Could you check a few things on this model? Use its own coordinates, in mm. A direction names the side the tool comes from. Round coordinates to 2 decimals unless told otherwise and drop trailing zeros. Write each loop counter-clockwise with the first axis right and the second up, starting at its lowest first coordinate (ties: lowest second). Pieces come first, ordered by that corner, then holes. Notation, with made-up numbers: (16, 15.5) -> (35, 15.5) arc R33 cw to (35, 51.5) -> close; hole circle Ø4 at (-30.75, 27.25). An arc over 180 degrees is marked (long way). Return JSON: item names as keys, results as strings.
Autodesk Fusion 360 part; units mm, degrees
sketch "Sketch1" plane through (0, 0, 0) normal (0, 0, 1) x (1, 0, 0)
  line L0 (25, 42.5) -> (-25, 42.5)
  line L1 (-25, 42.5) -> (-25, -42.5)
  line L2 (-25, -42.5) -> (25, -42.5)
  line L3 (25, -42.5) -> (25, 42.5)
  line L4 (25, 42.5) -> (-25, -42.5) construction
  line L5 (-25, 42.5) -> (25, -42.5) construction
  line L6 (25, 42.5) -> (46.6506, 55)
  line L7 (25, 42.5) -> (55, 42.5) construction
  line L8 (0, 42.5) -> (0, -42.5)
  line L9 (-25, 0) -> (25, 0)
  line L10 (25, 42.5) -> (23.5, 45.0981)
  line L11 (23.5, 45.0981) -> (45.1506, 57.5981)
  line L12 (45.1506, 57.5981) -> (46.6506, 55)
  line L13 (25, 42.5) -> (26.5, 39.9019)
  line L14 (26.5, 39.9019) -> (48.1506, 52.4019)
  line L15 (23.5, 45.0981) -> (19, 42.5)
  line L16 (26.5, 39.9019) -> (25, 39.0359)
  line L17 (48.1506, 52.4019) -> (46.6506, 55)
  circle A0 centre (46.6506, 55) radius 8.75
  circle A1 centre (46.6506, 55) radius 7.75
  line L18 (46.6506, 55) -> (42.7756, 61.7117)
  line L19 (46.6506, 55) -> (53.3623, 58.875)
  line L20 (46.6506, 55) -> (50.5256, 48.2883)
  circle A2 centre (46.6506, 55) radius 1.5
  line L21 (46.6506, 55) -> (50.9808, 57.5)
  circle A3 centre (50.9808, 57.5) radius 1.1
  circle A4 centre (42.3205, 52.5) radius 1.1
  line L22 (46.6506, 55) -> (44.1506, 59.3301)
  circle A5 centre (44.1506, 59.3301) radius 1.1
  circle A6 centre (49.1506, 50.6699) radius 1.1
  circle A7 centre (-49.1506, 50.6699) radius 1.1
  circle A8 centre (-50.9808, 57.5) radius 1.1
  circle A9 centre (-44.1506, 59.3301) radius 1.1
  circle A10 centre (-46.6506, 55) radius 1.5
  circle A11 centre (-42.3205, 52.5) radius 1.1
  line L23 (-23.5, 45.0981) -> (-45.1506, 57.5981)
  line L24 (-26.5, 39.9019) -> (-48.1506, 52.4019)
  circle A12 centre (-46.6506, 55) radius 8.75
  circle A13 centre (-46.6506, 55) radius 7.75
  line L25 (-26.5, 39.9019) -> (-25, 39.0359)
  line L26 (-23.5, 45.0981) -> (-19, 42.5)
  circle A14 centre (-46.6506, -55) radius 7.75
  circle A15 centre (-44.1506, -59.3301) radius 1.1
  circle A16 centre (-46.6506, -55) radius 1.5
  circle A17 centre (-49.1506, -50.6699) radius 1.1
  circle A18 centre (-42.3205, -52.5) radius 1.1
  circle A19 centre (-50.9808, -57.5) radius 1.1
  line L27 (-26.5, -39.9019) -> (-48.1506, -52.4019)
  line L28 (-23.5, -45.0981) -> (-45.1506, -57.5981)
  line L29 (-23.5, -45.0981) -> (-19, -42.5)
  line L30 (-26.5, -39.9019) -> (-25, -39.0359)
  line L31 (23.5, -45.0981) -> (19, -42.5)
  line L32 (26.5, -39.9019) -> (25, -39.0359)
  line L33 (26.5, -39.9019) -> (48.1506, -52.4019)
  line L34 (23.5, -45.0981) -> (45.1506, -57.5981)
  circle A20 centre (46.6506, -55) radius 8.75
  circle A21 centre (46.6506, -55) radius 7.75
  circle A22 centre (49.1506, -50.6699) radius 1.1
  circle A23 centre (46.6506, -55) radius 1.5
  circle A24 centre (42.3205, -52.5) radius 1.1
  circle A25 centre (44.1506, -59.3301) radius 1.1
  circle A26 centre (50.9808, -57.5) radius 1.1
  circle A27 centre (-46.6506, -55) radius 7.75
  circle A28 centre (-46.6506, -55) radius 8.75
  line L35 (25, 0) -> (25, -42.5)
  line L36 (0, 0) -> (0, -9)
  line L37 (0, -9) -> (0, -10.6)
  line L38 (0, -9) -> (0, -7.4)
  line L39 (0, -9) -> (1, -9)
  line L40 (19, -42.5) -> (25.9282, -46.5)
  line L41 (25, -39.0359) -> (25.0866, -34.0366)
  line L42 (19, -42.5) -> (16, -42.5)
  line L43 (19, -42.5) -> (14.6699, -40)
  line L44 (14.6699, -40) -> (34.8771, -40) construction
  line L45 (25, -39.0359) -> (17.5453, -34.8631)
  line L46 (14.6699, -40) -> (17.5453, -34.8631)
  line L47 (17.5453, -34.8631) -> (25, -21.5453)
  line L48 (25, -42.5) -> (25, -33)
  line L49 (25, -33) -> (15.5, -33)
  circle A29 centre (15.5, -33) radius 2.3
  circle A30 centre (15.5, -33) radius 4
  line L50 (-25, -42.5) -> (-18, -42.5)
  line L51 (-18, -42.5) -> (-18, -27.5)
  line L52 (-18, 42.5) -> (-18, 27.5)
  line L53 (-25, 42.5) -> (-18, 42.5)
  line L54 (18, 42.5) -> (18, 27.5)
  line L55 (18, -42.5) -> (18, -27.5)
  line L56 (18, -30) -> (18, 27.5)
  line L57 (18, 27.5) -> (-18, 27.5)
  line L58 (-18, 27.5) -> (-18, -27.5)
  line L59 (18, -27.5) -> (-18, -27.5)
  circle A31 centre (15.5, -33) radius 1.25
  circle A32 centre (-15.5, -33) radius 1.25
  circle A33 centre (-15.5, -33) radius 2.3
  circle A34 centre (-15.5, -33) radius 4
  circle A35 centre (-15.5, 33) radius 4
  circle A36 centre (-15.5, 33) radius 2.3
  circle A37 centre (-15.5, 33) radius 1.25
  circle A38 centre (15.5, 33) radius 1.25
  circle A39 centre (15.5, 33) radius 2.3
  circle A40 centre (15.5, 33) radius 4
  line L60 (18, 27.5) -> (18, 15.5)
  line L61 (18, 15.5) -> (-18, 15.5)
  line L62 (18, 15.5) -> (18, 10.5)
  line L63 (18, 10.5) -> (-18, 10.5)
  line L64 (18, -10.5) -> (-18, -10.5)
  line L65 (18, -15.5) -> (-18, -15.5)
  line L66 (0, 0) -> (0, 2.5)
  line L67 (0, 2.5) -> (-18, 2.5)
  line L68 (0, 2.5) -> (18, 2.5)
  line L69 (0, -2.5) -> (18, -2.5)
  line L70 (0, -2.5) -> (-18, -2.5)
  line L71 (0, 27.5) -> (10, 27.5)
  line L72 (10, 27.5) -> (10, 42.5)
  line L73 (-10, 27.5) -> (-10, 42.5)
  line L74 (10, 42.5) -> (10, 35.5)
  line L75 (10, 35.5) -> (-10, 35.5)
  line L76 (10, -35.5) -> (-10, -35.5)
  line L77 (-10, -27.5) -> (-10, -42.5)
  line L78 (10, -27.5) -> (10, -42.5)
  point P0 (-46.6506, -55)
  dimension "d1" = 50
  dimension "d2" = 85
  dimension "d4" = 25
  dimension "d5" = 30
  dimension "d6" = 3
  dimension "d7" = 25
  dimension "d8" = 17.5
  dimension "d9" = 15.5
  dimension "d10" = 3
  dimension "d11" = 5
  dimension "d12" = 2.2
  dimension "d13" = 5
  dimension "d14" = 2.2
  dimension "d23" = 9
  dimension "d24" = 1.6
  dimension "d25" = 1.6
  dimension "d51" = 8
  dimension "d76" = 5
  dimension "d77" = 3
  dimension "d88" = 5
  dimension "d130" = 180
  dimension "d131" = 9.5
  dimension "d132" = 9.5
  dimension "d133" = 4.6
  dimension "d134" = 8
  dimension "d141" = 7
  dimension "d142" = 15
  dimension "d170" = 2.5
  dimension "d180" = 12
  dimension "d181" = 5
  dimension "d182" = 2.5
  dimension "d186" = 10
  dimension "d187" = 7
extrude "Extrude1" add sketch "Sketch1" along normal blind 2 contours L3 L9 L35 L47 A30 L55 L56 | L3 L35 L47 L49 A30 | L8 L9 L36 L56 L69 | L8 L9 L56 L66 L68 | L3 L35 L45 L48 L49 A30 | L47 L49 A30 | L47 L49 A30 L55 L56 | L8 L36 L37 L38 L56 L64 L69 | L2 L3 L35 L43 L45 L48 A30 L55 | L45 L47 L49 A30 L55 | L47 L49 L55 | L46 L47 A30 L55 L56 | L2 L42 L43 L46 A30 L55 L56 L59 L78 | L8 L37 L56 L64 L65 | L45 A30 L55 | L45 L47 L55 | L43 L46 A30 L55 | L45 L46 A30 L55 | L8 L56 L59 L65 | L2 L42 L43 L55 | L8 L59 L76 L78 | L2 L8 L76 L78
extrude "Extrude3" add sketch "Sketch1" along normal blind 24 contours L47 L49 A30 | L47 L49 A30 L55 L56 | L45 L47 L49 A30 L55 | L47 L49 L55 | A29 | L46 L47 A30 L55 L56 | L45 A30 L55 | L45 L47 L55 | L45 L46 A30 L55
mirror "Mirror3" about plane through (0, -27.5, 0) normal (-1, 0, 0) of bodies 1 merged
extrude "Extrude6" cut sketch "Sketch1" along normal blind 12 contours L8 L36 L37 L38 L56 L64 L69 | L8 L56 L63 L68 | L8 L56 L57 L60 L61 L71 | L8 L58 L63 L67 | L8 L36 L37 L38 L58 L64 L70 | L8 L56 L61 L62 L63 | L8 L57 L58 L61 | L8 L56 L59 L65 | L8 L58 L61 L63 | L8 L58 L59 L65
fillet "Fillet4" radius 8 2 edges at (25, -42.5, 1) (-25, -42.5, 1)
mirror "Mirror5" about plane through (18, 0, 0) normal (0, 1, 0) of bodies 1 merged
fillet "Fillet8" radius 4 4 edges at (18, 27.5, 1) (-18, 27.5, 1) (18, -27.5, 1) (-18, -27.5, 1)
fillet "Fillet9" radius 4 12 edges at (-18, -15.5, 1) (-18, -10.5, 1) (-18, -2.5, 1) (-18, 2.5, 1) (18, 2.5, 1) (18, -2.5, 1) (18, -10.5, 1) (18, -15.5, 1) (18, 10.5, 1) (-18, 10.5, 1) (-18, 15.5, 1) (18, 15.5, 1)
chamfer "Chamfer46" distance 1 angle 45 4 edges at (11.7707, 31.5535, 2) (-11.7707, 31.5535, 2) (11.7707, -31.5535, 2) (-11.7707, -31.5535, 2)
extrude "Extrude9" cut sketch "Sketch1" along normal blind 7 contours L8 L57 L71 L72 L75 | L8 L57 L73 L75 | L8 L59 L76 L78 | L8 L59 L76 L77
fillet "Fillet10" radius 4 4 edges at (-10, -35.5, 1) (10, -35.5, 1) (10, 35.5, 1) (-10, 35.5, 1)
fillet "Fillet11" radius 4 4 edges at (-10, 27.5, 1) (10, 27.5, 1) (-10, -27.5, 1) (10, -27.5, 1)
1) I want a section at B-B, the plane y = -33. Please give me the cut outline in (x, z).
Return value:
{"outline": "(-25, 0) -> (-16.75, 0) -> (-16.75, 24) -> (-19.5, 24) -> (-19.5, 3) -> (-20.5, 2) -> (-25, 2) -> close; (-14.25, 0) -> (-9.71, 0) -> (-9.71, 2) -> (-10.5, 2) -> (-11.5, 3) -> (-11.5, 24) -> (-14.25, 24) -> close; (9.71, 0) -> (14.25, 0) -> (14.25, 24) -> (11.5, 24) -> (11.5, 3) -> (10.5, 2) -> (9.71, 2) -> close; (16.75, 0) -> (25, 0) -> (25, 2) -> (20.5, 2) -> (19.5, 3) -> (19.5, 24) -> (16.75, 24) -> close"}
2) I want a section at A-A, the plane z = 20.75. Please give me the cut outline in (x, y).
Return value:
{"outline": "circle Ø8 at (-15.5, -33); circle Ø8 at (-15.5, 33); circle Ø8 at (15.5, -33); circle Ø8 at (15.5, 33); hole circle Ø2.5 at (-15.5, -33); hole circle Ø2.5 at (-15.5, 33); hole circle Ø2.5 at (15.5, -33); hole circle Ø2.5 at (15.5, 33)"}
3) I want a section at D-D, the plane x = -15.5. Count the separate pieces of the cut face and the enclosed holes in it, and give its area (3 significant figures).
Return value:
{"separate pieces": "7", "enclosed holes": "0", "area": "329 mm²"}
4) Will these pins go through, and if not, where does the flat tip stop? pin 1 Ø6 at (x, y) = (-8, 20.5) entering from -Z; pin 2 Ø5 at (x, y) = (18.5, 29) entering from -Z; pin 3 Ø2 at (x, z) = (-12, 16) entering from -Y.
Return value:
{"pin 1": "through", "pin 2": "z = 0", "pin 3": "y = -36.12"}
5) Thinking about a two-plate mould opening in Y: for faces 3 (the face through (0, 42.5, 1)), 4 (the face through (0, -42.5, 1)), 5 (the face through (-16.797, 26.359, 1.014)), which applies, pulls with the +Y half, pulls with the -Y half, needs draft (parallel to the pull), parting line crosses it, or undercut?
Return value:
{"face 3": "pulls with the +Y half", "face 4": "pulls with the -Y half", "face 5": "undercut"}
6) For faces 1 (the face through (-16.86, 16.703, 1.014)), 2 (the face through (17, -33, 24)), which set-ups out of +Z, -Z, +X, -X, +Y, -Y let a thin tool reach every point of the face, with its end or its side?
Return value:
{"face 1": "+Z, -Z", "face 2": "+Z, +X, -X, +Y, -Y"}
7) I want a section at C-C, the plane x = -9. Please give me the cut outline in (y, z).
Return value:
{"outline": "(-42.5, 0) -> (-34.15, 0) -> (-34.15, 2) -> (-42.5, 2) -> close; (-15.5, 0) -> (-10.5, 0) -> (-10.5, 2) -> (-15.5, 2) -> close; (-2.5, 0) -> (2.5, 0) -> (2.5, 2) -> (-2.5, 2) -> close; (10.5, 0) -> (15.5, 0) -> (15.5, 2) -> (10.5, 2) -> close; (34.15, 0) -> (42.5, 0) -> (42.5, 2) -> (34.15, 2) -> close"}
8) If I drill on probe 1 along Y at (x, z) = (15.5, 7); probe 2 along Y at (x, z) = (-16, 15.25); probe 3 along Z at (x, y) = (2, 36), over which ranges is the centre line in solid material (lowest first)? Write a range as [from, to].
Return value:
{"probe 1": "[-37, -34.25], [-31.75, -29], [29, 31.75], [34.25, 37]", "probe 2": "[-36.97, -34.15], [-31.85, -29.03], [29.03, 31.85], [34.15, 36.97]", "probe 3": "[0, 2]"}
